from build123d import *

# Parameters (mm, degrees)
CROQUIS1_R                 = 5.5
SALIENTE_EXTRUIR1_DEPTH    = 26.5
CROQUIS2_R                 = 7.2
SALIENTE_EXTRUIR2_DEPTH    = 2.3
CROQUIS3_W                 = 11.5
CROQUIS3_H                 = 4.45
SALIENTE_EXTRUIR3_DEPTH    = 14
CORTAR_EXTRUIR1_DEPTH      = 13.37
CROQUIS6_R                 = 4
CORTAR_EXTRUIR2_DEPTH      = 26.5
CROQUIS7_R                 = 2.8
CORTAR_EXTRUIR3_DEPTH      = 26.37
CHAFL_N1_SIZE              = 0.9
CHAFL_N1_SIZE2             = 3.358845727
CHAFL_N2_SIZE              = 3.358845727
CHAFL_N2_SIZE_2            = 0.9
REDONDEO1_R                = 0.2
REDONDEO2_R                = 0.2
CROQUIS11_W                = 4
CROQUIS11_H                = 22.3
CORTAR_EXTRUIR4_DEPTH      = 48.550085436
CORTAR_EXTRUIR5_DEPTH      = 8.4
REDONDEO3_R                = 0.2
CROQUIS14_W                = 14.4
CROQUIS14_H                = 26.5
CORTAR_EXTRUIR6_DEPTH      = 28.4
SALIENTE_EXTRUIR4_DEPTH    = 3.4
SALIENTE_EXTRUIR5_DEPTH    = 22.5
SALIENTE_EXTRUIR6_DEPTH    = 4.2
CHAFL_N3_SIZE              = 1
CHAFL_N3_SIZE2             = 0.577350269
S_LIDO_MOVER_COPIAR1_ANGLE = 90


with BuildPart() as part:
    # Croquis1 → Saliente-Extruir1 (new body)
    with BuildSketch(Plane(origin=(0, 0, 0), x_dir=(1, 0, 0), z_dir=(0, 1, 0))):
        with Locations(Location((0, 0, 0), (0, 0, 270))):
            Circle(CROQUIS1_R)
    extrude(amount=SALIENTE_EXTRUIR1_DEPTH)

    # Croquis2 → Saliente-Extruir2 (add)
    with BuildSketch(Plane(origin=(0, 26.5, 0), x_dir=(1, 0, 0), z_dir=(0, 1, 0))):
        with Locations(Location((0, 0, 0), (0, 0, 270))):
            Circle(CROQUIS2_R)
    extrude(amount=SALIENTE_EXTRUIR2_DEPTH)

    # Croquis3 → Saliente-Extruir3 (add)
    with BuildSketch(Plane(origin=(0, 28.8, 0), x_dir=(1, 0, 0), z_dir=(0, 1, 0))):
        Rectangle(CROQUIS3_W, CROQUIS3_H)
    extrude(amount=SALIENTE_EXTRUIR3_DEPTH)

    # Croquis4 → Cortar-Extruir1 (cut)
    with BuildSketch(Plane.XY.offset(2.225)):
        with BuildLine():
            Line((5.75, 42.8), (0, 42.8))
            ThreePointArc((0, 42.8), (4.065863992, 41.115863992), (5.75, 37.05))
            Line((5.75, 37.05), (5.75, 42.8))
        make_face()
        with BuildLine():
            Line((0, 42.8), (-5.75, 42.8))
            Line((-5.75, 42.8), (-5.75, 37.05))
            ThreePointArc((-5.75, 37.05), (-4.065863992, 41.115863992), (0, 42.8))
        make_face()
    extrude(amount=-CORTAR_EXTRUIR1_DEPTH, mode=Mode.SUBTRACT)

    # Croquis6 → Cortar-Extruir2 (cut)
    with BuildSketch(Plane.XZ):
        with Locations(Location((0, 0, 0), (0, 0, 270))):
            Circle(CROQUIS6_R)
    extrude(amount=-CORTAR_EXTRUIR2_DEPTH, mode=Mode.SUBTRACT)

    # Croquis7 → Cortar-Extruir3 (cut)
    with BuildSketch(Plane.XY.offset(2.225)):
        with Locations((0, 37.05)):
            Circle(CROQUIS7_R)
    extrude(amount=-CORTAR_EXTRUIR3_DEPTH, mode=Mode.SUBTRACT)

    # Chaflán1
    chafl_n1_edges = [part.edges().sort_by_distance(p)[0] for p in [
        (-2.8, 37.05, 2.225),
    ]]
    chafl_n1_side = [part.faces().sort_by_distance(p)[0] for p in [
        (0, 28.981176709, 2.225),
    ]]
    chamfer(chafl_n1_edges, length=CHAFL_N1_SIZE, length2=CHAFL_N1_SIZE2, reference=chafl_n1_side[0])

    # Chaflán2
    # the kernel refuses this chamfer: 3.358845727, 0.9 mm, written as the material it takes off along each edge
    with BuildSketch(Plane(origin=(0, 37.05, -2.225), x_dir=(1, 0, 0), z_dir=(0, -1, 0))) as chafl_n2_piece_1:
        Polygon((2.8, CHAFL_N2_SIZE), (2.8 + CHAFL_N2_SIZE_2, 0), (2.8, 0), align=None)
    revolve(axis=Axis((0, 37.05, -2.225), (0, 0, 1)), mode=Mode.SUBTRACT)

    # Redondeo1
    redondeo1_edges = [part.edges().sort_by_distance(p)[0] for p in [
        (-5.75, 32.925, 2.225),
        (-5.75, 32.925, -2.225),
        (0, 42.8, 2.225),
        (0, 42.8, -2.225),
        (5.75, 32.925, -2.225),
        (5.75, 32.925, 2.225),
    ]]
    fillet(redondeo1_edges, radius=REDONDEO1_R)

    # Redondeo2
    redondeo2_edges = [part.edges().sort_by_distance(p)[0] for p in [
        (-3.7, 37.05, 2.225),
        (-3.7, 37.05, -2.225),
        (-3.103813047, 37.05, 0),
    ]]
    fillet(redondeo2_edges, radius=REDONDEO2_R)

    # Croquis11 → Cortar-Extruir4 (cut, through all)
    with BuildSketch(Plane.XY.offset(12.225)):
        with Locations((0, 15.35)):
            Rectangle(CROQUIS11_W, CROQUIS11_H)
    extrude(amount=-CORTAR_EXTRUIR4_DEPTH, mode=Mode.SUBTRACT)

    # Croquis13 → Cortar-Extruir5 (cut)
    with BuildSketch(Plane.XZ):
        with BuildLine():
            Line((-2, -4.19791615), (4.520060123, 1.091584394))
            ThreePointArc((4.520060123, 1.091584394), (3.611110666, 2.929569892), (2, 4.19791615))
            Line((2, 4.19791615), (-4.520060123, -1.091584394))
            ThreePointArc((-4.520060123, -1.091584394), (-3.611110666, -2.929569892), (-2, -4.19791615))
        make_face()
    extrude(amount=-CORTAR_EXTRUIR5_DEPTH, mode=Mode.SUBTRACT)

    # Redondeo3
    redondeo3_edges = [part.edges().sort_by_distance(p)[0] for p in [
        (-2, 4.2, -4.660695766),
        (-2, 4.2, 4.293788499),
        (-2, 26.5, -4.293788499),
        (-2, 26.5, 4.293788499),
        (2, 26.5, 4.293788499),
        (2, 26.5, -4.293788499),
        (2, 4.2, -4.293788499),
        (2, 4.2, 4.660695766),
    ]]
    fillet(redondeo3_edges, radius=REDONDEO3_R)

    # Croquis14 → Cortar-Extruir6 (cut)
    with BuildSketch(Plane(origin=(15.75, 0, 0), x_dir=(0, 0, -1), z_dir=(1, 0, 0))):
        with Locations((0, 13.25)):
            Rectangle(CROQUIS14_W, CROQUIS14_H)
    extrude(amount=-CORTAR_EXTRUIR6_DEPTH, mode=Mode.SUBTRACT)

    # Chaflán3
    chafl_n3_edges = [part.edges().sort_by_distance(p)[0] for p in [
        (0, 28.8, -7.2),
    ]]
    chafl_n3_side = [part.faces().sort_by_distance(p)[0] for p in [
        (-5.953646753, 28.8, 0),
    ]]
    chamfer(chafl_n3_edges, length=CHAFL_N3_SIZE, length2=CHAFL_N3_SIZE2, reference=chafl_n3_side[0])


with BuildPart() as body_2:
    # Croquis15 → Saliente-Extruir4 (new body)
    with BuildSketch(Plane.XZ.offset(-26.5)):
        with BuildLine():
            Line((-1.3, 5.395600059), (-1.3, 1.3))
            Line((-1.3, 1.3), (-5.395600059, 1.3))
            ThreePointArc((-5.395600059, 1.3), (-5.55, 0), (-5.395600059, -1.3))
            Line((-5.395600059, -1.3), (-1.3, -1.3))
            Line((-1.3, -1.3), (-1.3, -5.395600059))
            ThreePointArc((-1.3, -5.395600059), (0, -5.55), (1.3, -5.395600059))
            Line((1.3, -5.395600059), (1.3, -1.3))
            Line((1.3, -1.3), (5.395600059, -1.3))
            ThreePointArc((5.395600059, -1.3), (5.55, 0), (5.395600059, 1.3))
            Line((5.395600059, 1.3), (1.3, 1.3))
            Line((1.3, 1.3), (1.3, 5.395600059))
            ThreePointArc((1.3, 5.395600059), (0, 5.55), (-1.3, 5.395600059))
        make_face()
    extrude(amount=SALIENTE_EXTRUIR4_DEPTH)


with BuildPart() as body_3:
    # Croquis16 → Saliente-Extruir5 (new body)
    with BuildSketch(Plane.XZ.offset(-23.1)):
        with BuildLine():
            Line((-3.623879137, 1.3), (-1.3, 1.3))
            Line((-1.3, 1.3), (-1.3, 3.623879137))
            ThreePointArc((-1.3, 3.623879137), (0, 3.85), (1.3, 3.623879137))
            Line((1.3, 3.623879137), (1.3, 1.3))
            Line((1.3, 1.3), (3.623879137, 1.3))
            ThreePointArc((3.623879137, 1.3), (3.85, 0), (3.623879137, -1.3))
            Line((3.623879137, -1.3), (1.3, -1.3))
            Line((1.3, -1.3), (1.3, -3.623879137))
            ThreePointArc((1.3, -3.623879137), (0, -3.85), (-1.3, -3.623879137))
            Line((-1.3, -3.623879137), (-1.3, -1.3))
            Line((-1.3, -1.3), (-3.623879137, -1.3))
            ThreePointArc((-3.623879137, -1.3), (-3.85, 0), (-3.623879137, 1.3))
        make_face()
    extrude(amount=SALIENTE_EXTRUIR5_DEPTH)


with BuildPart() as body_4:
    # Croquis17 → Saliente-Extruir6 (new body)
    with BuildSketch(Plane.XZ.offset(-0.6)):
        with BuildLine():
            Line((-3.45, 1.3), (3.45, 1.3))
            ThreePointArc((3.45, 1.3), (4.75, 0), (3.45, -1.3))
            Line((3.45, -1.3), (-3.45, -1.3))
            ThreePointArc((-3.45, -1.3), (-4.75, 0), (-3.45, 1.3))
        make_face()
    extrude(amount=-SALIENTE_EXTRUIR6_DEPTH)


with BuildPart() as body_3_1:
    add(body_3.part)

    # Combinar1: union body 4
    add(body_4.part)


with BuildPart() as body_2_1:
    add(body_2.part)

    # Combinar2: union body 3
    add(body_3_1.part)


with BuildPart() as body_2_2:
    # Sólido-Mover/Copiar1: moved
    add(body_2_1.part.rotate(Axis((0, 0, 0), (0, 1, 0)), S_LIDO_MOVER_COPIAR1_ANGLE))

    # Combinar3: union part
    add(part.part)


solid = body_2_2.part
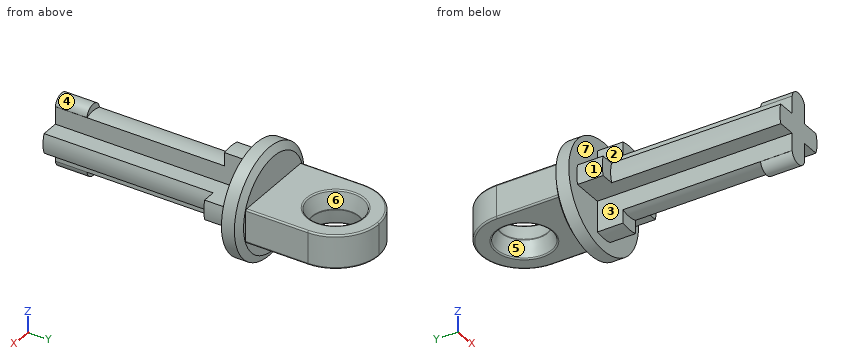
Part model, mm, in its own coordinate system. Face numbers are marked on the shaded views. A direction names the side the tool comes from. Coordinates: 2 decimals unless noted, no trailing zeros. Loops run counter-clockwise (first coordinate to the right, second up) from the corner with the lowest first, then second, coordinate; pieces in that order, holes last. Notation, with made-up numbers: (62, -23) -> (93, -23) arc R29 ccw to (93, -2) -> close; hole circle Ø11 at (85.5, 20). An arc over 180 degrees is marked (long way). Use a Markdown table: item, result. Add a question column.
Item 1: Which spindle directions (+Z, -Z, +X, -X, +Y, -Y) get a long thin tool onto all of the face, cutting with end or side? Do the marked faces 1, 2 and 3. Say none if no direction does.
Item 2: Band-saw the part on B-B on y = 13. Write the cut outline in (x, z), plus the area to 3 significant figures.
Item 3: Band-saw the part on A-A on y = 30. Write the cut outline in (x, z) (3 decimals).
Item 4: Band-saw the part on C-C on y = 25.5. Write the cut outline in (x, z).
Item 5: Probe probe 1 along Y at (x, z) = (1, -3.75); probe 2 along Y at (x, z) = (1.75, 5.5); probe 3 along Z at (x, y) = (-2.5, 33) (3 decimals). List the from-to ranges inside material, lowest first.
Item 6: Flat gauge pins, fed straight in: P1, Ø2, axis at y = 12, z = 2.5, coming from the +X side; P2, Ø5, axis at x = -3.5, z = -3, coming from the -Y side; P3, Ø5, axis at x = 5, z = 4, coming from the -Y side; P4, Ø4.5, axis at y = 32, z = -1, coming from the +X side. Where does each tip first touch, or does it go through?
Item 7: Pull direction X, two halves, no side cores. Call the marked faces 4, 5, 6 and 7: +X half, -X half, draft (parallel to the pull), parting line (faces both ways), or undercut.
Geometry says:
| question | item | result |
|---|---|---|
| 1 | face 1 | -X, -Y |
| 1 | face 2 | +Z, -X, -Y |
| 1 | face 3 | -Z, -X, -Y |
| 2 | outline | (-3.62, -1.3) -> (-1.3, -1.3) -> (-1.3, -3.62) arc R3.85 ccw to (1.3, -3.62) -> (1.3, -1.3) -> (3.62, -1.3) arc R3.85 ccw to (3.62, 1.3) -> (1.3, 1.3) -> (1.3, 3.62) arc R3.85 ccw to (-1.3, 3.62) -> (-1.3, 1.3) -> (-3.62, 1.3) arc R3.85 ccw to start |
| 2 | area | 32.5 mm² |
| 3 | outline | (-5.75, -2.025) arc R0.2 ccw to (-5.55, -2.225) -> (5.55, -2.225) arc R0.2 ccw to (5.75, -2.025) -> (5.75, 2.025) arc R0.2 ccw to (5.55, 2.225) -> (-5.55, 2.225) arc R0.2 ccw to (-5.75, 2.025) -> close |
| 4 | outline | (-5.4, -1.3) -> (-1.3, -1.3) -> (-1.3, -5.4) arc R5.55 ccw to (1.3, -5.4) -> (1.3, -1.3) -> (5.4, -1.3) arc R5.55 ccw to (5.4, 1.3) -> (1.3, 1.3) -> (1.3, 5.4) arc R5.55 ccw to (-1.3, 5.4) -> (-1.3, 1.3) -> (-5.4, 1.3) arc R5.55 ccw to start |
| 5 | probe 1 | 0.6 to 4.8, 23.1 to 28.8 |
| 5 | probe 2 | 26.5 to 28.8 |
| 5 | probe 3 | -2.225 to 2.225 |
| 6 | P1 | x = 1.3 |
| 6 | P2 | y = 0.6 |
| 6 | P3 | y = 26.5 |
| 6 | P4 | x = 5.75 |
| 7 | face 4 | parting line |
| 7 | face 5 | undercut |
| 7 | face 6 | undercut |
| 7 | face 7 | draft |
